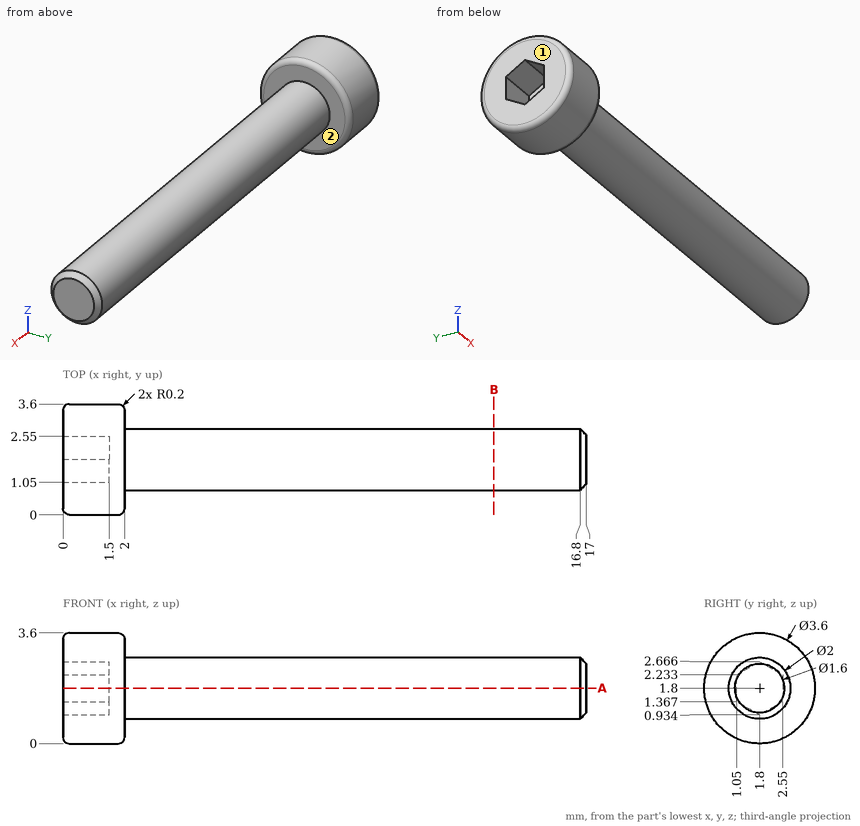
For this review, use the dimensioned drawing (mm, ordinates from the lowest corner) and the shaded views. A direction names the side the tool comes from. Round coordinates to 2 decimals unless told otherwise and drop trailing zeros. Write each loop counter-clockwise with the first axis right and the second up, starting at its lowest first coordinate (ties: lowest second). Pieces come first, ordered by that corner, then holes. Notation, with made-up numbers: M 65.5,88 L 113.5,88 A24 cw 113.5,101 Z; hole C -5,78 d3. An arc over 180 degrees is marked long. Write item = value, one per line. Start each with the question number.
(1) We need section B-B (x = 14). Give the boundary of the cut face in (y, z).
(2) For line 1 along X through (y, z) = (2, 0.25); line 2 along X through (y, z) = (2.3, 1.7); line 3 along Z through (x, y) = (6.25, 1.75), list the stretches that pass through material, from the lowest coordinate up.
(3) Clearance check with flat-ended pins moving along their axes: pin 1 Ø1 at (x, y) = (10.5, 1.5) entering from +Z; pin 2 Ø1.5 at (x, z) = (12.5, 2) entering from -Y. State where each tip first meets the part, or that it passes through.
(4) For the marked faces 1 and 2, list the 3-axis set-ups (+Z, -Z, +X, -X, +Y, -Y) from which the entire face can be reached by the end or side of a thin tool; tool diameter is ignored.
(5) We need section A-A (z = 1.8). Give the boundary of the cut face in (x, y), then the cut area to 3 significant figures.
Results found:
q1.outline = C 1.8,1.8 d2
q2.line_1 = 0 to 2
q2.line_2 = 1.5 to 17
q2.line_3 = 0.8 to 2.8
q3.pin_1 = 2.8
q3.pin_2 = 0.8
q4.face_1 = +Z, -Z, -X, +Y, -Y
q4.face_2 = +X
q5.outline = M 0,0.2 A0.2 ccw 0.2,0 L 1.8,0 A0.2 ccw 2,0.2 L 2,0.8 L 16.8,0.8 L 17,1 L 17,2.6 L 16.8,2.8 L 2,2.8 L 2,3.4 A0.2 ccw 1.8,3.6 L 0.2,3.6 A0.2 ccw 0,3.4 L 0,2.55 L 1.5,2.55 L 1.5,1.05 L 0,1.05 Z
q5.area = 34.9 mm²
